```python
from build123d import *

# Parameters (mm, degrees)
SKETCH_W     = 7.45
SKETCH_H     = 11.35
PAD_DEPTH    = 9.5
SKETCH001_W  = 0.8
SKETCH001_H  = 9.5
PAD001_DEPTH = 0.01
SKETCH005_W  = 0.8
SKETCH005_H  = 2
PAD004_DEPTH = 0.8
SKETCH006_W  = 1
SKETCH006_H  = 0.7
PAD005_DEPTH = 3.5
SKETCH002_R  = 3
PAD002_DEPTH = 15
SKETCH003_W  = 3.35
SKETCH003_H  = 9.5
POCKET_DEPTH = 7
SKETCH004_R  = 3.25
PAD003_DEPTH = 5
SKETCH007_W  = 1
SKETCH007_H  = 1
PAD006_DEPTH = 2
SKETCH008_R  = 0.5
PAD007_DEPTH = 4.5


with BuildPart() as pad001:
    # Sketch → Pad (new body)
    with BuildSketch(Plane.XZ):
        with Locations((0.130678, -0.133685)):
            Rectangle(SKETCH_W, SKETCH_H)
    extrude(amount=PAD_DEPTH)

    # Sketch001 → Pad001 (new body)
    with BuildSketch(Plane(origin=(3.855678, 0, 0), x_dir=(0, 0, 1), z_dir=(1, 0, 0))):
        with Locations((-5.408685, 4.75)):
            Rectangle(SKETCH001_W, SKETCH001_H)
    extrude(amount=PAD001_DEPTH)


with BuildPart() as pad005:
    # Pad004 base: copy of Pad001
    add(pad001.part)

    # Sketch005 → Pad004 (new body)
    with BuildSketch(Plane(origin=(3.865678, 0, 0), x_dir=(0, 0, 1), z_dir=(1, 0, 0))):
        with Locations((-5.408685, 4.75)):
            Rectangle(SKETCH005_W, SKETCH005_H)
    extrude(amount=PAD004_DEPTH)

    # Sketch006 → Pad005 (new body)
    with BuildSketch(Plane(origin=(-3.594322, 0, 0), x_dir=(0, 0, -1), z_dir=(-1, 0, 0))):
        with Locations((-0.191315, 9.75)):
            Rectangle(SKETCH006_W, SKETCH006_H)
        with Locations((-0.191315, -0.25)):
            Rectangle(SKETCH006_W, SKETCH006_H)
    extrude(amount=PAD005_DEPTH)


with BuildPart() as fusion:
    # Pad002 base: copy of Pad001
    add(pad001.part)

    # Sketch002 → Pad002 (new body)
    with BuildSketch(Plane(origin=(3.855678, 0, 0), x_dir=(0, 0, 1), z_dir=(1, 0, 0))):
        with Locations((0.691315, 4.75)):
            Circle(SKETCH002_R)
    extrude(amount=PAD002_DEPTH)

    # Sketch003 → Pocket (cut)
    with BuildSketch(Plane(origin=(18.855678, 0, 0), x_dir=(0, 0, 1), z_dir=(1, 0, 0))):
        with Locations((3.866315, 4.75)):
            Rectangle(SKETCH003_W, SKETCH003_H)
    extrude(amount=-POCKET_DEPTH, mode=Mode.SUBTRACT)

    # Sketch004 → Pad003 (new body)
    with BuildSketch(Plane(origin=(3.855678, 0, 0), x_dir=(0, 0, 1), z_dir=(1, 0, 0))):
        with Locations((0.691315, 4.75)):
            Circle(SKETCH004_R)
    extrude(amount=PAD003_DEPTH)

    # Sketch007 → Pad006 (new body)
    with BuildSketch(Plane(origin=(0, 0, -5.808685), x_dir=(1, 0, 0), z_dir=(0, 0, -1))):
        with Locations((-2.094322, 7.375)):
            Rectangle(SKETCH007_W, SKETCH007_H)
        with Locations((-2.094322, 4.75)):
            Rectangle(SKETCH007_W, SKETCH007_H)
        with Locations((-2.094322, 2.125)):
            Rectangle(SKETCH007_W, SKETCH007_H)
    extrude(amount=PAD006_DEPTH)

    # Sketch008 → Pad007 (new body)
    with BuildSketch(Plane(origin=(-2.594322, 0, 0), x_dir=(0, 0, -1), z_dir=(-1, 0, 0))):
        with Locations((7.308685, 4.75)):
            Circle(SKETCH008_R)
        with Locations((7.308685, 7.375)):
            Circle(SKETCH008_R)
        with Locations((7.308685, 2.125)):
            Circle(SKETCH008_R)
    extrude(amount=PAD007_DEPTH)

    # Fusion: union Pad005
    add(pad005.part)


solid = fusion.part
```
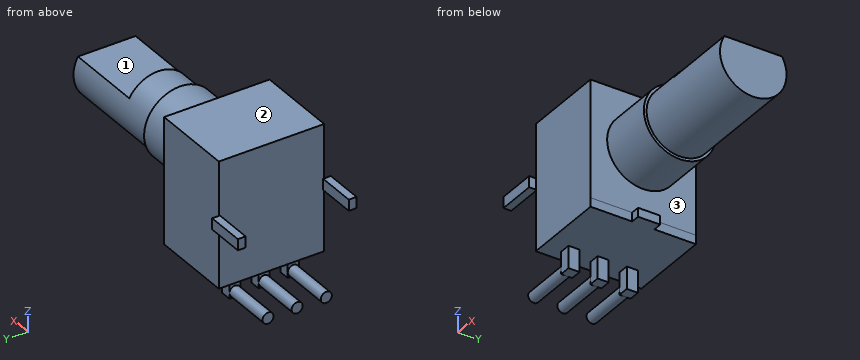
Input: part model. Units: mm. Frame: model coordinates. Face numbers are marked on the shaded views. A direction names the side the tool comes from. Round coordinates to 2 decimals unless told otherwise and drop trailing zeros. Loops run counter-clockwise (first coordinate to the right, second up) from the corner with the lowest first, then second, coordinate; pieces in that order, holes last. Notation, with made-up numbers: M 59.5,67 L 68.5,67 A13 ccw 68.5,92 Z; hole C 23.5,-27 d8. An arc over 180 degrees is marked long. Answer in a Markdown table with one row per item. Add a question column.
1. Section D-D (x = 7.25). Output: boundary loops of the cut face in (y, z).
2. Section C-C (z = 4.25). Output: boundary loops of the cut face in (x, y), and give its area (3 significant figures).
3. Set-up query: the marked faces 1, 2 and 3. Return all of +Z, -Z, +X, -X, +Y, -Y with unobstructed straight access to the full face (end or side cutting, diameter ignored); none if empty.
4. Ray query, probe 1 along X at (y, z) = (-6.75, 2.5); probe 2 along X at (y, z) = (-1.25, -4.25); probe 3 along Y at (x, z) = (1.25, -1.5). Return the intervals inside material, ascending.
5. Section A-A (x = 1.5). Output: boundary loops of the cut face in (y, z), and give its area (3 significant figures).
6. Contact query for flat-ended pins moving along their axis: pin 1 (3 mm diameter, centred on y = -4, z = -0.5, fed in from -X); pin 2 (1.2 mm diameter, centred on y = -4, z = 3, fed in from +X); pin 3 (5.5 mm diameter, centred on x = 13.5, y = -4.5, fed in from +Z). Output: stop coordinate, or through.
Values follow:
| question | item | result |
|---|---|---|
| 1 | outline | C -4.75,0.69 d6.5 |
| 2 | outline | M -3.59,-9.5 L 3.86,-9.5 L 3.86,0 L -3.59,0 Z |
| 2 | area | 70.8 mm^2 |
| 3 | face 1 | +Z, +X, +Y, -Y |
| 3 | face 2 | +Z, +X, -X, +Y, -Y |
| 3 | face 3 | +X |
| 4 | probe 1 | -3.59 to 11.86 |
| 4 | probe 2 | -3.59 to 3.86 |
| 4 | probe 3 | -9.5 to 0 |
| 5 | outline | M -9.5,-5.81 L 0,-5.81 L 0,5.54 L -9.5,5.54 Z |
| 5 | area | 108 mm^2 |
| 6 | pin 1 | x = -3.59 |
| 6 | pin 2 | x = 11.86 |
| 6 | pin 3 | z = 3.69 |
